from build123d import *

# Parameters (mm, degrees)
BOSS_EXTRUDE1_DEPTH = 40
SKETCH3_W           = 42
SKETCH3_H           = 42
SKETCH3_W_2         = 40
SKETCH3_H_2         = 40
CUT_EXTRUDE2_DEPTH  = 2


with BuildPart() as part:
    # Sketch1 → Boss-Extrude1 (new body)
    with BuildSketch(Plane(origin=(0, 0, 0), x_dir=(1, 0, 0), z_dir=(0, 1, 0))):
        with BuildLine():
            ThreePointArc((-17, 20), (-17.878679656, 17.878679656), (-20, 17))
            Line((-20, 17), (-30, 17))
            Line((-30, 17), (-30, -17))
            Line((-30, -17), (-20, -17))
            ThreePointArc((-20, -17), (-17.878679656, -17.878679656), (-17, -20))
            Line((-17, -20), (-17, -30))
            Line((-17, -30), (17, -30))
            Line((17, -30), (17, -20))
            ThreePointArc((17, -20), (17.878679656, -17.878679656), (20, -17))
            Line((20, -17), (30, -17))
            Line((30, -17), (30, 17))
            Line((30, 17), (20, 17))
            ThreePointArc((20, 17), (17.878679656, 17.878679656), (17, 20))
            Line((17, 20), (17, 30))
            Line((17, 30), (-17, 30))
            Line((-17, 30), (-17, 20))
        make_face()
    extrude(amount=BOSS_EXTRUDE1_DEPTH)

    # Sketch3 → Cut-Extrude2 (cut)
    with BuildSketch(Plane(origin=(0, 40, 0), x_dir=(1, 0, 0), z_dir=(0, 1, 0))):
        Rectangle(SKETCH3_W, SKETCH3_H)
        Rectangle(SKETCH3_W_2, SKETCH3_H_2, mode=Mode.SUBTRACT)
    extrude(amount=-CUT_EXTRUDE2_DEPTH, mode=Mode.SUBTRACT)


solid = part.part
Geometry: final body of the model. Coordinates: model frame, mm. A direction names the side the tool comes from. Give positions to 0.01 mm unless a question says otherwise; leave off trailing zeros. Write each loop counter-clockwise with the first axis right and the second up, starting at its lowest first coordinate (ties: lowest second). Pieces come first, ordered by that corner, then holes.
(1) Access query for faces 1 (the flat face through (-17, 20, 25)), 2 (the flat face through (21, 39, 0)), 3 (the flat face through (0, 39, -21)), 4 (the flat face through (25, 20, 17)). Directions: +Z, -Z, +X, -X, +Y, -Y. A direction counts if a zero-diameter tool reaches every point of the face in a straight line with its end or side. Return the directions, or none.
(2) Cut plane B-B, the plane x = -25.5. Return loops of the section in (y, z), then the cut area to 3 significant figures.
(3) Cut plane A-A, the plane y = 32. Return loops of the section in (x, z), then the cut area to 3 significant figures.
(4) First-contact query: P1, Ø8, axis at x = 23, y = 20.5, coming from the -Z side; P2, Ø8, axis at y = 11, z = 27, coming from the +X side; P3, Ø0.5, axis at x = -8, z = -20.5, coming from the +Y side. Flat tips, straight axial feed; report the tip coordinate or a pass-through.
(5) Mould query, pull axis Z, two halves, no side actions, for faces 5 (the flat face through (0, 39, 20)), 6 (the cylindrical face through (-17.86, 19.72, -17.9)), 7 (the flat face through (0, 0, 0)). Classes: released by +Z, released by -Z, zero draft, split by the parting line, or undercut.
(6) Ray query, line 1 (X direction, y = 37, z = -22.5); line 2 (Z direction, x = -18, y = 37.5). Return the intervals inside material, ascending.
(7) Cut plane C-C, the plane z = -23.5. Return loops of the section in (x, y).
Values follow:
1. face 1: +Z, -X, +Y, -Y
1. face 2: +Z, -Z, +Y
1. face 3: +X, -X, +Y
1. face 4: +Z, +X, +Y, -Y
2. outline: (0, -17) - (40, -17) - (40, 17) - (0, 17) - close
2. area: 1,360 mm2
3. outline: (-30, -17) - (-20, -17) arc R3 cw to (-17, -20) - (-17, -30) - (17, -30) - (17, -20) arc R3 cw to (20, -17) - (30, -17) - (30, 17) - (20, 17) arc R3 cw to (17, 20) - (17, 30) - (-17, 30) - (-17, 20) arc R3 cw to (-20, 17) - (-30, 17) - close
3. area: 2,930 mm2
4. P1: stops at z = -17.17
4. P2: stops at x = 17
4. P3: stops at y = 38
5. face 5: undercut
5. face 6: released by -Z
5. face 7: zero draft
6. line 1: x = -17 to 17
6. line 2: z = -17.76 to 17.76
7. outline: (-17, 0) - (17, 0) - (17, 40) - (-17, 40) - close
